Verification items for the finished model (mm, model axes). A direction names the side the tool comes from. Coordinates: 2 decimals unless noted, no trailing zeros. Write each loop counter-clockwise with the first axis right and the second up, starting at its lowest first coordinate (ties: lowest second). Pieces come first, ordered by that corner, then holes.
```python
from build123d import *

# Parameters (mm, degrees)
SKETCH1_W           = 190
SKETCH1_H           = 190
SKETCH1_R           = 20
SKETCH1_R_2         = 5
SKETCH1_W_2         = 44
SKETCH1_H_2         = 44
BOSS_EXTRUDE2_DEPTH = 20
SKETCH2_R           = 20
SKETCH2_R_2         = 6
BOSS_EXTRUDE5_DEPTH = 50
SKETCH4_R           = 20
BOSS_EXTRUDE6_DEPTH = 3
FILLET1_R           = 10
SKETCH6_W           = 60
SKETCH6_H           = 60
SKETCH6_W_2         = 44
SKETCH6_H_2         = 44
BOSS_EXTRUDE7_DEPTH = 80


with BuildPart() as part:
    # Sketch1 → Boss-Extrude2 (new body)
    with BuildSketch(Plane.XY):
        Rectangle(SKETCH1_W, SKETCH1_H)
        with Locations((-70, 0)):
            Circle(SKETCH1_R, mode=Mode.SUBTRACT)
        with Locations((70, 0)):
            Circle(SKETCH1_R, mode=Mode.SUBTRACT)
        with Locations((70, -68.596885854)):
            Circle(SKETCH1_R_2, mode=Mode.SUBTRACT)
        with Locations((-70, -73.596885854)):
            Circle(SKETCH1_R_2, mode=Mode.SUBTRACT)
        with Locations((70, 73.936439664)):
            Circle(SKETCH1_R_2, mode=Mode.SUBTRACT)
        with Locations((-70, 78.936439664)):
            Circle(SKETCH1_R_2, mode=Mode.SUBTRACT)
        Rectangle(SKETCH1_W_2, SKETCH1_H_2, mode=Mode.SUBTRACT)
    extrude(amount=BOSS_EXTRUDE2_DEPTH)

    # Sketch2 → Boss-Extrude5 (add)
    with BuildSketch(Plane.XY):
        with Locations((-70, 0)):
            Circle(SKETCH2_R)
        with Locations((-70, 0)):
            Circle(SKETCH2_R_2, mode=Mode.SUBTRACT)
        with Locations((70, 0)):
            Circle(SKETCH2_R)
        with Locations((70, 0)):
            Circle(SKETCH2_R_2, mode=Mode.SUBTRACT)
    extrude(amount=BOSS_EXTRUDE5_DEPTH)

    # Sketch4 → Boss-Extrude6 (add)
    with BuildSketch(Plane.XY):
        with Locations((70, 0)):
            Circle(SKETCH4_R)
        with Locations((-70, 0)):
            Circle(SKETCH4_R)
    extrude(amount=BOSS_EXTRUDE6_DEPTH)

    # Fillet1
    fillet1_edges = [part.edges().sort_by_distance(p)[0] for p in [
        (95, -95, 10),
        (-95, -95, 10),
        (-95, 95, 10),
        (95, 95, 10),
    ]]
    fillet(fillet1_edges, radius=FILLET1_R)

    # Sketch6 → Boss-Extrude7 (add)
    with BuildSketch(Plane.XY):
        Rectangle(SKETCH6_W, SKETCH6_H)
        Rectangle(SKETCH6_W_2, SKETCH6_H_2, mode=Mode.SUBTRACT)
    extrude(amount=BOSS_EXTRUDE7_DEPTH)


solid = part.part
```
1. Sectioned sample at D-D, the plane z = 17.5. Record the boundary of the cut face in (x, y), and give its area (3 significant figures).
2. Gauge pin test, flat ends, axial feed: P1, Ø16, axis at x = 70, y = -68.6, coming from the +Z side; P2, Ø13, axis at x = -2.5, z = 41.5, coming from the +Y side; P3, Ø11, axis at x = -70, y = 0, coming from the +Z side; P4, Ø6, axis at x = -70, y = 78.94, coming from the -Z side. Record the tip position at first contact, or that the pin passes through.
3. Sectioned sample at B-B, the plane z = 67.5. Record the boundary of the cut face in (x, y).
4. Material ranges on L1, parallel to Y at x = -70, z = 7; L2, parallel to Y at x = 8, z = 28; L3, parallel to Y at x = -68.5, z = 9.5, recorded low to high.
5. Draft check along X on faces 1 (the cylindrical face through (91.99, -92.15, 10.14)), 2 (the flat face through (-1, -95, 10)), 3 (the cylindrical face through (50.02, 0.88, 34.79)), 4 (the cylindrical face through (-65.23, 80.44, 9.86)). Enter one of: pulls with the +X half, pulls with the -X half, needs draft (parallel to the pull), parting line crosses it, or undercut.
6. Sectioned sample at C-C, the plane y = 0. Record the boundary of the cut face in (x, z).
7. Tool access check on faces 5 (the flat face through (-30, 0, 50)), 6 (the flat face through (-75, -4, 50)), 7 (the flat face through (0, -22, 39)), 8 (the cylindrical face through (-76, 0, 26)), 9 (the flat face through (65, -4, 50)). Record the directions out of +Z, -Z, +X, -X, +Y, -Y that give a thin tool (end or side, any length) a straight path to the whole face; none if there is none.
8. Sectioned sample at A-A, the plane x = -70. Record the boundary of the cut face in (y, z), and give its area (3 significant figures).
Outcome:
1. outline: (-95, -85) arc R10 ccw to (-85, -95) - (85, -95) arc R10 ccw to (95, -85) - (95, 85) arc R10 ccw to (85, 95) - (-85, 95) arc R10 ccw to (-95, 85) - close; hole circle Ø12 at (-70, 0); hole circle Ø10 at (-70, -73.6); hole circle Ø10 at (-70, 78.94); hole (-22, -22) - (22, -22) - (22, 22) - (-22, 22) - close; hole circle Ø12 at (70, 0); hole circle Ø10 at (70, -68.6); hole circle Ø10 at (70, 73.94)
1. area: 33,500 mm2
2. P1: stops at z = 20
2. P2: stops at y = 30
2. P3: stops at z = 3
2. P4: passes through
3. outline: (-30, -30) - (30, -30) - (30, 30) - (-30, 30) - close; hole (-22, -22) - (22, -22) - (22, 22) - (-22, 22) - close
4. L1: y = -95 to -78.6, -68.6 to -6, 6 to 73.94, 83.94 to 95
4. L2: y = -30 to -22, 22 to 30
4. L3: y = -95 to -78.37, -68.83 to -5.81, 5.81 to 74.17, 83.71 to 95
5. face 1: pulls with the +X half
5. face 2: needs draft
5. face 3: undercut
5. face 4: undercut
6. outline: (-95, 0) - (-22, 0) - (-22, 80) - (-30, 80) - (-30, 20) - (-50, 20) - (-50, 50) - (-64, 50) - (-64, 3) - (-76, 3) - (-76, 50) - (-90, 50) - (-90, 20) - (-95, 20) - close; (22, 0) - (95, 0) - (95, 20) - (90, 20) - (90, 50) - (76, 50) - (76, 3) - (64, 3) - (64, 50) - (50, 50) - (50, 20) - (30, 20) - (30, 80) - (22, 80) - close
7. face 5: +Z, +Y, -Y
7. face 6: +Z, -X, +Y, -Y
7. face 7: +Z, -Z
7. face 8: +Z
7. face 9: +Z, +X, +Y, -Y
8. outline: (-95, 0) - (-78.6, 0) - (-78.6, 20) - (-95, 20) - close; (-68.6, 0) - (73.94, 0) - (73.94, 20) - (20, 20) - (20, 50) - (6, 50) - (6, 3) - (-6, 3) - (-6, 50) - (-20, 50) - (-20, 20) - (-68.6, 20) - close; (83.94, 0) - (95, 0) - (95, 20) - (83.94, 20) - close
8. area: 4,040 mm2
